from build123d import *

# Parameters (mm, degrees)
CROQUIS1_R              = 17.7
SALIENTE_EXTRUIR1_DEPTH = 60.4
REDONDEO1_R             = 6
REDONDEO2_R             = 2
CROQUIS2_R              = 8.25
SALIENTE_EXTRUIR2_DEPTH = 16.5
CROQUIS3_R              = 0.5
SALIENTE_EXTRUIR3_DEPTH = 9


with BuildPart() as part:
    # Croquis1 → Saliente-Extruir1 (new body)
    with BuildSketch(Plane(origin=(0, 0, 0), x_dir=(1, 0, 0), z_dir=(0, 1, 0))):
        Circle(CROQUIS1_R)
    extrude(amount=SALIENTE_EXTRUIR1_DEPTH)

    # Redondeo1
    redondeo1_edges = [part.edges().sort_by_distance(p)[0] for p in [
        (-17.7, 60.4, 0),
    ]]
    fillet(redondeo1_edges, radius=REDONDEO1_R)

    # Redondeo2
    redondeo2_edges = [part.edges().sort_by_distance(p)[0] for p in [
        (-17.7, 0, 0),
    ]]
    fillet(redondeo2_edges, radius=REDONDEO2_R)

    # Croquis2 → Saliente-Extruir2 (add)
    with BuildSketch(Plane(origin=(0, 60.4, 0), x_dir=(1, 0, 0), z_dir=(0, 1, 0))):
        Circle(CROQUIS2_R)
    extrude(amount=SALIENTE_EXTRUIR2_DEPTH)

    # Croquis3 → Saliente-Extruir3 (add)
    with BuildSketch(Plane(origin=(0, 76.9, 0), x_dir=(1, 0, 0), z_dir=(0, 1, 0))):
        Circle(CROQUIS3_R)
    extrude(amount=SALIENTE_EXTRUIR3_DEPTH)


solid = part.part
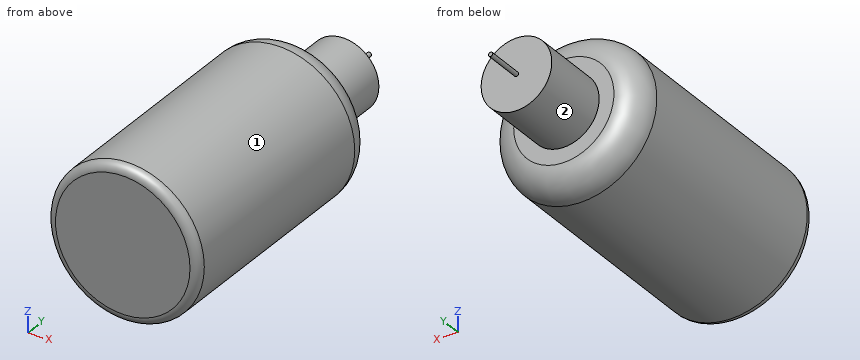
Part model, mm, in its own coordinate system. Face numbers are marked on the shaded views. A direction names the side the tool comes from. Give positions to 0.01 mm unless a question says otherwise; leave off trailing zeros. Order: outer loops, then holes, each group sorted by start corner. A loop starts at its lowest first (then second) coordinate and runs counter-clockwise, first axis right, second up. Notation, with made-up numbers: (-17.5, 27.25) - (3.5, 27.25) arc R9 ccw to (3.5, 44.25) - close; hole circle Ø2 at (-6.75, 8). An arc over 180 degrees is marked (long way). Use a Markdown table: item, result.
1) Probe L1, parallel to Y at x = -0.5, z = -11.5; L2, parallel to Y at x = 2, z = 6.5; L3, parallel to X at y = 59.5, z = 9. List the from-to ranges inside material, lowest first. Write a range as from..to.
Checked values:
| item | result |
|---|---|
| L1 | 0..60.4 |
| L2 | 0..76.9 |
| L3 | -11.83..11.83 |
2) Saw through at A-A on y = 78.5. List the corners of the cut face in (x, z).
Checked values:
| item | result |
|---|---|
| outline | circle Ø1 at (0, 0) |
3) Saw through at B-B on y = 68. List the corners of the cut face in (x, z), plus the area to 3 significant figures.
Checked values:
| item | result |
|---|---|
| outline | circle Ø16.5 at (0, 0) |
| area | 214 mm² |
4) Flat gauge pins, fed straight in: P1, Ø1.5, axis at x = -7.5, y = 55, coming from the -Z side; P2, Ø4, axis at x = -9, y = 75.5, coming from the -Z side; P3, Ø5, axis at y = 42.5, z = -8, coming from the +X side. Where does each tip first touch, or does it go through?
Checked values:
| item | result |
|---|---|
| P1 | z = -16.34 |
| P2 | z = -4.37 |
| P3 | x = 16.82 |
5) 3-axis set-ups, long thin cutter, end or side, ignore diameter. For the marked faces 1 and 2: which of +Z, -Z, +X, -X, +Y, -Y reach the whole face in a straight line?
Checked values:
| item | result |
|---|---|
| face 1 | +Y, -Y |
| face 2 | +Y |
